```python
from build123d import *

# Parameters (mm, degrees)
RESSALTO_EXTRUS_O12_DEPTH = 6.7
ESBO_O7_R                 = 1.15
CORTE_EXTRUS_O3_DEPTH     = 6.7


with BuildPart() as part:
    # Esboço4 → Ressalto-extrusão12 (new body)
    with BuildSketch(Plane(origin=(0, 0, 0), x_dir=(0, 0, -1), z_dir=(1, 0, 0))):
        with BuildLine():
            Line((0, 0), (0, 1.65))
            ThreePointArc((0, 1.65), (0.175735931, 2.074264069), (0.6, 2.25))
            Line((0.6, 2.25), (8.101, 2.25))
            ThreePointArc((8.101, 2.25), (8.171710678, 2.220710678), (8.201, 2.15))
            Line((8.201, 2.15), (8.201, 1.65))
            ThreePointArc((8.201, 1.65), (8.171710678, 1.579289322), (8.101, 1.55))
            Line((8.101, 1.55), (0.7, 1.55))
            Line((0.7, 1.55), (0.7, 0))
            Line((0.7, 0), (0, 0))
        make_face()
    extrude(amount=RESSALTO_EXTRUS_O12_DEPTH)

    # Esboço7 → Corte-extrusão3 (cut)
    with BuildSketch(Plane(origin=(0, 2.25, 0), x_dir=(1, 0, 0), z_dir=(0, 1, 0))):
        with Locations((3.35, 4.1005)):
            Circle(ESBO_O7_R)
    extrude(amount=-CORTE_EXTRUS_O3_DEPTH, mode=Mode.SUBTRACT)


solid = part.part
```
CAD build for the part. Positions are in the model's coordinates, mm. A direction names the side the tool comes from. Give positions to 0.01 mm unless a question says otherwise; leave off trailing zeros. Loops run counter-clockwise (first coordinate to the right, second up) from the corner with the lowest first, then second, coordinate; pieces in that order, holes last. Notation, with made-up numbers: (3, 5.5) - (57, 5.5) arc R14 ccw to (57, 20.5) - close; hole circle Ø7 at (-30, -9). An arc over 180 degrees is marked (long way). Put each result on its own line as item: value.
Q1. Probe line 1 along Z through (x, y) = (3.35, 1.7); line 2 along Z through (x, y) = (0.5, 1.5); line 3 along Y through (x, z) = (6.25, -3.5). List the from-to ranges inside material, lowest first.
Filled in:
line 1: z = -8.2 to -5.25, -2.95 to 0
line 2: z = -0.7 to 0
line 3: y = 1.55 to 2.25
Q2. Slice it at D-D (y = 1.4). Give the cut face in (x, z).
Filled in:
outline: (0, -0.7) - (6.7, -0.7) - (6.7, 0) - (0, 0) - close
Q3. Tool access for faces 5 (the face through (5, 2.25, -4)), 6 (the face through (3, 1, -0.7)): list every direction of +Z, -Z, +X, -X, +Y, -Y with a clear straight run to the whole face (end or side of a thin tool).
Filled in:
face 5: +Z, -Z, +X, -X, +Y
face 6: -Z, +X, -X, -Y
Q4. Mould opens along X. For faces 1 (the face through (3, 1, 0)), 2 (the face through (6.7, 2, -3)), 3 (the face through (0, 2, -3)), 4 (the face through (2.44, 1.9, -3.4)) say: pulls with the +X half, pulls with the -X half, needs draft (parallel to the pull), parting line crosses it, or undercut.
Filled in:
face 1: needs draft
face 2: pulls with the +X half
face 3: pulls with the -X half
face 4: undercut
Q5. Slice it at C-C (x = 5). Give the cut face in (y, z).
Filled in:
outline: (0, -0.7) - (1.55, -0.7) - (1.55, -8.1) arc R0.1 ccw to (1.65, -8.2) - (2.15, -8.2) arc R0.1 ccw to (2.25, -8.1) - (2.25, -0.6) arc R0.6 ccw to (1.65, 0) - (0, 0) - close
Q6. Slice it at B-B (z = -3.5). Give the cut face in (x, y), plus the area to 3 significant figures.
Filled in:
outline: (0, 1.55) - (2.37, 1.55) - (2.37, 2.25) - (0, 2.25) - close; (4.33, 1.55) - (6.7, 1.55) - (6.7, 2.25) - (4.33, 2.25) - close
area: 3.32 mm²
Q7. Slice it at A-A (x = 3.35). Give the cut face in (y, z), plus the area to 3 significant figures.
Filled in:
outline: (0, -0.7) - (1.55, -0.7) - (1.55, -2.95) - (2.25, -2.95) - (2.25, -0.6) arc R0.6 ccw to (1.65, 0) - (0, 0) - close; (1.55, -8.1) arc R0.1 ccw to (1.65, -8.2) - (2.15, -8.2) arc R0.1 ccw to (2.25, -8.1) - (2.25, -5.25) - (1.55, -5.25) - close
area: 5.13 mm²
Q8. Flat gauge pin, fed straight in: pin 1 (1.5 mm diameter, centred on x = 5, z = -5, fed in from -Y). Where does the tip first touch, or does it go through?
Filled in:
pin 1: stops at y = 1.55
